Build history of the part. All positions in model axes, mm. Face numbers are marked on the shaded views. A direction names the side the tool comes from. Give positions to 0.01 mm unless a question says otherwise; leave off trailing zeros. Order: outer loops, then holes, each group sorted by start corner. A loop starts at its lowest first (then second) coordinate and runs counter-clockwise, first axis right, second up. Notation, with made-up numbers: (48.5, -9.75) - (74.5, -9.75) arc R30 ccw to (74.5, 23.25) - close; hole circle Ø4 at (67, 21.5). An arc over 180 degrees is marked (long way). Use a Markdown table: item, result. Add a question column.
(1) Slice it at D-D (y = 1.5). Write the cut outline in (x, z), then the cut area to 3 significant figures.
(2) Slice it at B-B (y = -0.5). Write the cut outline in (x, z).
(3) Wall check: line 1 (Z direction, x = -13.75, y = -1.2); line 2 (X direction, y = -1.65, z = -0.1); line 3 (Y direction, x = -9, z = 3.5). Give the ranges that are in metal, low to high.
(4) Slice it at A-A (x = 10). Write the cut outline in (y, z), then the cut area to 3 significant figures.
(5) Mould opens along X. For the marked faces 1, 2, 3 and 4 say: +X half, -X half, draft (parallel to the pull), parting line (faces both ways), or undercut.
(6) Flat gauge pins, fed straight in: pin 1 (1.8 mm diameter, centred on x = -7.25, z = -0.1, fed in from +Y); pin 2 (6 mm diameter, centred on x = -12, z = 1.5, fed in from +Y); pin 3 (5 mm diameter, centred on x = 10, z = 0, fed in from -Y). Where does each tip first touch, or does it go through?
(7) Slice it at C-C (x = -7.25). Write the cut outline in (y, z).
(8) Which spindle directions (+Z, -Z, +X, -X, +Y, -Y) get a long thin tool onto all of the face, cutting with end or side? Do the marked faces 5 and 6. Say none if no direction does.
Autodesk Inventor part; units mm, degrees
ref_plane "YZ Plane" through (0, 0, 0) normal (1, 0, 0) x (0, 1, 0)
ref_plane "XZ Plane" through (0, 0, 0) normal (0, 1, 0) x (-1, 0, 0)
ref_plane "XY Plane" through (0, 0, 0) normal (0, 0, 1) x (1, 0, 0)
sketch "Sketch1" plane through (0, 0, 0) normal (0, 0, 1) x (1, 0, 0)
  line L0 (-17, 0) -> (0, 0)
  line L1 (-17, -4) -> (-17, 0)
  line L2 (0, 4) -> (20, 4)
  line L3 (20, 4) -> (20, -1)
  line L4 (20, -1) -> (2, -1)
  line L5 (0, 0) -> (0, 4)
  line L6 (0, -4) -> (0, 4) construction
  line L7 (-17, -4) -> (2, -4)
  line L8 (2, -4) -> (2, -1)
  line L9 (0, -4) -> (0, 4) construction
  line L10 (2, -4) -> (2, 4) construction
  point P0 (2, 0)
  dimension "d0" = 5
  dimension "d2" = 4
  dimension "d3" = 20
  dimension "d13" = 19
  dimension "d14" = 2
  dimension "d15" = 4
extrude "Extrusion1" add sketch "Sketch1" along normal mid plane 10
sketch "Sketch2" plane through (0, 4, 5) normal (0, 1, 0) x (1, 0, 0)
  circle A0 centre (10, 5) radius 2.1
  line L0 (20, 0) -> (20, 10)
  point P0 (0, 5)
  point P1 (20, 5)
  dimension "d7" = 4.2
  dimension "d8" = 10
extrude "Extrusion2" cut sketch "Sketch2" against normal through all
fillet "Fillet1" radius 2 4 edges at (0, 0, 0) (0, 4, 0) (2, -4, 0) (2, -1, 0)
sketch "Sketch3" plane through (-17, 0, 5) normal (0, 1, 0) x (1, 0, 0)
  circle A0 centre (9.75, 5.1) radius 1.15
  circle A1 centre (3.25, 5.1) radius 1.15
  line L0 (15, 0) -> (0, 0)
  line L1 (0, 10) -> (0, 0)
  point P0 (17, 5)
  dimension "d17" = 2.3
  dimension "d18" = 6.5
  dimension "d19" = 5.1
  dimension "d20" = 3.25
extrude "Extrusion3" cut sketch "Sketch3" against normal through all
fillet "Fillet2" radius 2 4 edges at (-17, -2, 5) (-17, -2, -5) (20, 1.5, -5) (20, 1.5, 5)
properties part number "y-endstop-bracket"
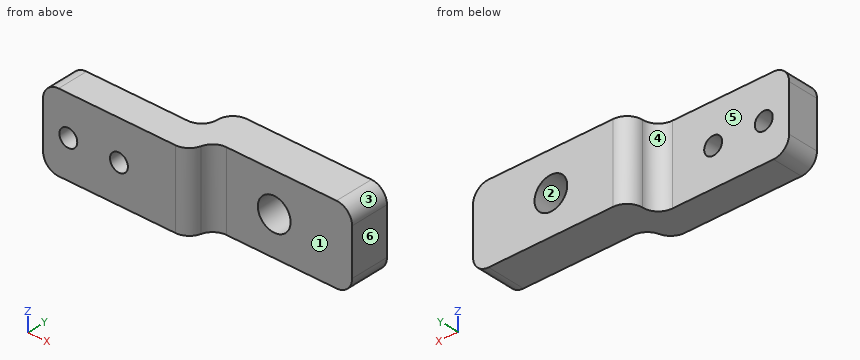
Solution:
| question | item | result |
|---|---|---|
| 1 | outline | (-0.06, -5) - (18, -5) arc R2 ccw to (20, -3) - (20, 3) arc R2 ccw to (18, 5) - (-0.06, 5) - close; hole circle Ø4.2 at (10, 0) |
| 1 | area | 185 mm2 |
| 2 | outline | (-17, -3) arc R2 ccw to (-15, -5) - (18, -5) arc R2 ccw to (20, -3) - (20, 3) arc R2 ccw to (18, 5) - (-15, 5) arc R2 ccw to (-17, 3) - close; hole circle Ø2.3 at (-13.75, -0.1); hole circle Ø2.3 at (-7.25, -0.1); hole circle Ø4.2 at (10, 0) |
| 3 | line 1 | -5 to -1.25, 1.05 to 5 |
| 3 | line 2 | -17 to -14.9, -12.6 to -8.4, -6.1 to 2.4 |
| 3 | line 3 | -4 to 0 |
| 4 | outline | (-1, -5) - (4, -5) - (4, -2.1) - (-1, -2.1) - close; (-1, 2.1) - (4, 2.1) - (4, 5) - (-1, 5) - close |
| 4 | area | 29.0 mm2 |
| 5 | face 1 | draft |
| 5 | face 2 | undercut |
| 5 | face 3 | +X half |
| 5 | face 4 | -X half |
| 6 | pin 1 | through |
| 6 | pin 2 | y = 0 |
| 6 | pin 3 | y = -1 |
| 7 | outline | (-4, -5) - (0, -5) - (0, -1.25) - (-4, -1.25) - close; (-4, 1.05) - (0, 1.05) - (0, 5) - (-4, 5) - close |
| 8 | face 5 | +Z, -Z, -X, +Y |
| 8 | face 6 | +Z, -Z, +X, +Y, -Y |
